Print and shaded views of the part. All mm, measured from the part's lowest x, y and z. A direction names the side the tool comes from. Round coordinates to 2 decimals unless told otherwise and drop trailing zeros. Loops run counter-clockwise (first coordinate to the right, second up) from the corner with the lowest first, then second, coordinate; pieces in that order, holes last. Notation, with made-up numbers: (-22.75, 81) -> (10.25, 81) arc R28 cw to (10.25, 118) -> close; hole circle Ø11 at (46, -18.75). An arc over 180 degrees is marked (long way). Use a Markdown table: item, result.
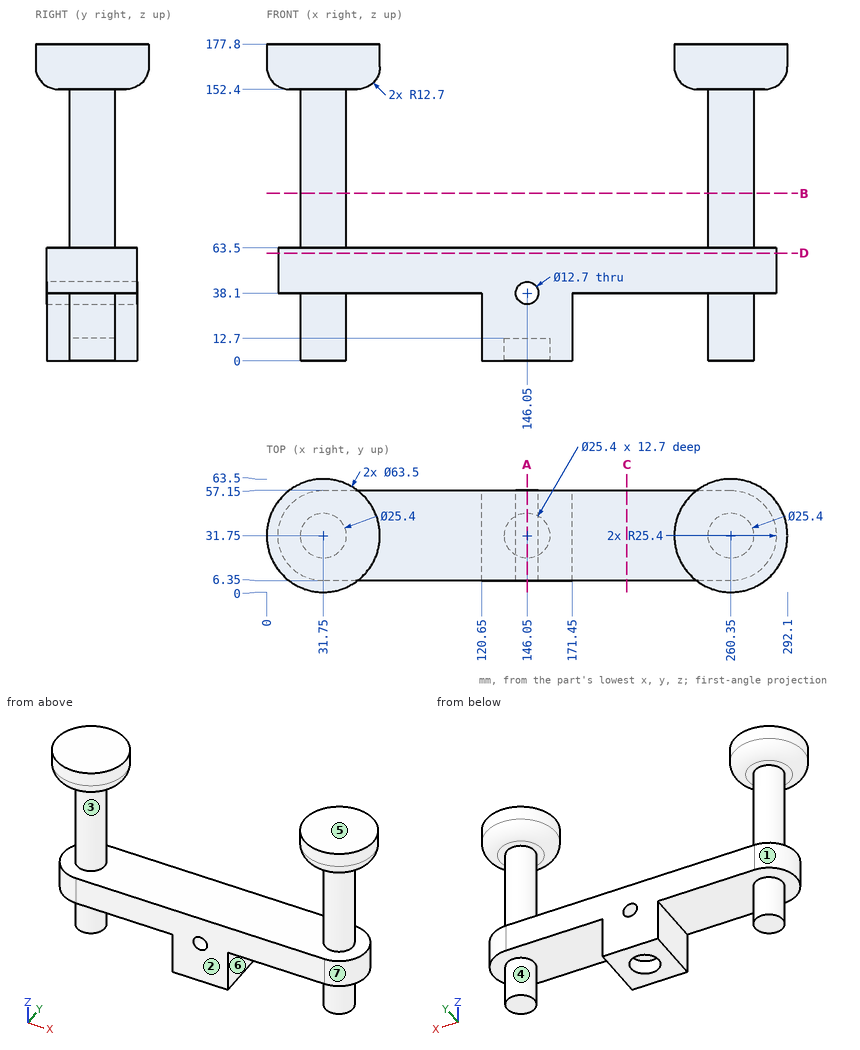
Q1. Tool access for the marked faces 1, 2, 3 and 4: list every direction of +Z, -Z, +X, -X, +Y, -Y with a clear straight run to the whole face (end or side of a thin tool).
Results list:
| item | result |
|---|---|
| face 1 | -Z, -X |
| face 2 | -Z, +X, -X, -Y |
| face 3 | none |
| face 4 | -Z |
Q2. Band-saw the part on A-A, the plane x = 146.05. Give the cut face in (y, z).
Results list:
| item | result |
|---|---|
| outline | (6.35, 0) -> (19.05, 0) -> (19.05, 12.7) -> (44.45, 12.7) -> (44.45, 0) -> (57.15, 0) -> (57.15, 31.75) -> (6.35, 31.75) -> close; (6.35, 44.45) -> (57.15, 44.45) -> (57.15, 63.5) -> (6.35, 63.5) -> close |
Q3. Pull direction X, two halves, no side cores. Call the marked faces 5, 6 and 7: released by +X, released by -X, zero draft, split by the parting line, or undercut.
Results list:
| item | result |
|---|---|
| face 5 | zero draft |
| face 6 | undercut |
| face 7 | released by +X |
Q4. Drill centre lines: L1, parallel to X at y = 33, z = 38; L2, parallel to Y at x = 146.05, z = 5.25; L3, parallel to Z at x = 33, y = 17. Where is each one in solid material? Low to high. Write a range as from..to.
Results list:
| item | result |
|---|---|
| L1 | x = 19.11..44.39, 120.65..139.7, 152.4..171.45, 247.71..272.99 |
| L2 | y = 6.35..19.05, 44.45..57.15 |
| L3 | z = 38.1..63.5, 152.4..177.8 |
Q5. Flat gauge pins, fed straight in: pin 1 (16.5 mm diameter, centred on x = 146.05, z = 38.1, fed in from -Y); pin 2 (5 mm diameter, centred on x = 88.5, y = 43.5, fed in from +Z); pin 3 (8 mm diameter, centred on x = 45.5, z = 152, fed in from -Y). Where does each tip first touch, or does it go through?
Results list:
| item | result |
|---|---|
| pin 1 | stops at y = 6.35 |
| pin 2 | stops at z = 63.5 |
| pin 3 | stops at y = 7.02 |
Q6. Band-saw the part on C-C, the plane x = 202. Give the cut face in (y, z), plus the area to 3 significant figures.
Results list:
| item | result |
|---|---|
| outline | (6.35, 38.1) -> (57.15, 38.1) -> (57.15, 63.5) -> (6.35, 63.5) -> close |
| area | 1,290 mm² |
Q7. Band-saw the part on D-D, the plane z = 60.5. Give the cut face in (x, y).
Results list:
| item | result |
|---|---|
| outline | (31.75, 6.35) -> (260.35, 6.35) arc R25.4 ccw to (260.35, 57.15) -> (31.75, 57.15) arc R25.4 ccw to start |
Q8. Band-saw the part on B-B, the plane z = 94. Give the cut face in (x, y).
Results list:
| item | result |
|---|---|
| outline | circle Ø25.4 at (31.75, 31.75); circle Ø25.4 at (260.35, 31.75) |
